```python
from build123d import *

# Parameters (mm, degrees)
SKETCH1_W           = 24.3
SKETCH1_H           = 12.9
BOSS_EXTRUDE1_DEPTH = 51.5
FILLET1_R           = 5
SHELL1_START        = 1.4
SHELL1_DEPTH        = 48.7
SKETCH2_W           = 18.539285396
SKETCH2_H           = 48.7
CUT_EXTRUDE1_DEPTH  = 5
SKETCH3_W           = 24.3
SKETCH3_H           = 4.6
SKETCH3_H_2         = 16.8
CUT_EXTRUDE2_DEPTH  = 5


# Read off the part's stored shape, not the designer's step: Shell1
with BuildPart() as part:
    # Sketch1 → Boss-Extrude1 (new body)
    with BuildSketch(Plane.XY):
        Rectangle(SKETCH1_W, SKETCH1_H)
    extrude(amount=BOSS_EXTRUDE1_DEPTH)

    # Fillet1
    fillet1_edges = [part.edges().sort_by_distance(p)[0] for p in [
        (-12.15, 6.45, 25.75),
        (12.15, 6.45, 25.75),
    ]]
    fillet(fillet1_edges, radius=FILLET1_R)

    # Shell1 outline → Shell1 (cut)
    with BuildSketch(Plane.XY.offset(SHELL1_START)):
        with BuildLine():
            Line((7.15, 5.05), (7.15, 6.45))
            Line((7.15, 6.45), (-7.15, 6.45))
            Line((-7.15, 6.45), (-7.15, 5.05))
            ThreePointArc((-7.15, 5.05), (-9.695584412, 3.995584412), (-10.75, 1.45))
            Line((-10.75, 1.45), (-10.75, -5.05))
            Line((-10.75, -5.05), (10.75, -5.05))
            Line((10.75, -5.05), (10.75, 1.45))
            ThreePointArc((10.75, 1.45), (9.695584412, 3.995584412), (7.15, 5.05))
        make_face()
    extrude(amount=SHELL1_DEPTH, mode=Mode.SUBTRACT)

    # Sketch2 → Cut-Extrude1 (cut)
    with BuildSketch(Plane(origin=(0, 6.45, 0), x_dir=(1, 0, 0), z_dir=(0, 1, 0))):
        with Locations((0, -25.75)):
            Rectangle(SKETCH2_W, SKETCH2_H)
    extrude(amount=-CUT_EXTRUDE1_DEPTH, mode=Mode.SUBTRACT)

    # Sketch3 → Cut-Extrude2 (cut)
    with BuildSketch(Plane(origin=(0, 6.45, 0), x_dir=(1, 0, 0), z_dir=(0, 1, 0))):
        with Locations((0, -3.7)):
            Rectangle(SKETCH3_W, SKETCH3_H)
        with Locations((0, -47.8)):
            Rectangle(SKETCH3_W, SKETCH3_H)
        with Locations((0, -25.75)):
            Rectangle(SKETCH3_W, SKETCH3_H_2)
    extrude(amount=-CUT_EXTRUDE2_DEPTH, mode=Mode.SUBTRACT)


solid = part.part
```
Here's how the part is built. I have some questions about the finished solid (model axes, mm). A direction names the side the tool comes from. Coordinates: 2 decimals unless noted, no trailing zeros. Order: outer loops, then holes, each group sorted by start corner. A loop starts at its lowest first (then second) coordinate and runs counter-clockwise, first axis right, second up.
Item 1: If we section it at B-B, the plane z = 19: List the corners of the cut face in (x, y) for me, then the cut area to 3 significant figures.
Response values:
outline: (-12.15, -6.45) - (12.15, -6.45) - (12.15, 1.45) - (10.75, 1.45) - (10.75, -5.05) - (-10.75, -5.05) - (-10.75, 1.45) - (-12.15, 1.45) - close
area: 52.2 mm2
Item 2: If we section it at A-A, the plane y = -1: List the corners of the cut face in (x, z) for me, then the cut area to 3 significant figures.
Response values:
outline: (-12.15, 0) - (12.15, 0) - (12.15, 51.5) - (-12.15, 51.5) - close; hole (-10.75, 1.4) - (10.75, 1.4) - (10.75, 50.1) - (-10.75, 50.1) - close
area: 204 mm2
Item 3: If we section it at D-D, the plane x = 3.5: List the corners of the cut face in (y, z) for me, then the cut area to 3 significant figures.
Response values:
outline: (-6.45, 0) - (6.45, 0) - (6.45, 1.4) - (-5.05, 1.4) - (-5.05, 50.1) - (6.45, 50.1) - (6.45, 51.5) - (-6.45, 51.5) - close
area: 104 mm2
Item 4: Which directions (+Z, -Z, +X, -X, +Y, -Y) give clear straight access to the entire face, cutting with the end or side of a thin tool? Please do faces 5 (the face through (9.27, 5, 40)), 6 (the face through (11.39, 4.1, 11.75)), 7 (the face through (10.75, -2, 25)), 8 (the face through (11, 4, 6)).
Response values:
face 5: +Y
face 6: +Z, -Z, +X, +Y
face 7: none
face 8: +X, -X, +Y
Item 5: I'm going to push flat-ended pins straight in: pin 1 Ø1 at (x, z) = (-9, 37.5) entering from +Y; pin 2 Ø5 at (y, z) = (4.5, 26) entering from +X; pin 3 Ø1.5 at (x, z) = (11.5, 3.5) entering from +Y; pin 4 Ø10 at (x, z) = (-4.5, 23) entering from +Y. Where does each tip first touch, or does it pass through?
Response values:
pin 1: stops at y = 5.98
pin 2: passes through
pin 3: stops at y = 1.45
pin 4: stops at y = -5.05
Item 6: I need wall thicknesses on probe 1 along Z at (x, y) = (10.5, 3.75); probe 2 along Z at (x, y) = (-9.25, -3.75); probe 3 along X at (y, z) = (-1, 40). Which ranges of each line are inside material? Lowest first, please.
Response values:
probe 1: z = 0 to 1.4, 6 to 17.35, 34.15 to 45.5, 50.1 to 51.5
probe 2: z = 0 to 1.4, 50.1 to 51.5
probe 3: x = -12.15 to -10.75, 10.75 to 12.15
Item 7: If we section it at C-C, the plane y = 3.5: List the corners of the cut face in (x, z) for me, then the cut area to 3 significant figures.
Response values:
outline: (-11.71, 0) - (11.71, 0) - (11.71, 1.4) - (-11.71, 1.4) - close; (-11.71, 6) - (-10.11, 6) - (-10.11, 17.35) - (-11.71, 17.35) - close; (-11.71, 34.15) - (-10.11, 34.15) - (-10.11, 45.5) - (-11.71, 45.5) - close; (-11.71, 50.1) - (11.71, 50.1) - (11.71, 51.5) - (-11.71, 51.5) - close; (10.11, 6) - (11.71, 6) - (11.71, 17.35) - (10.11, 17.35) - close; (10.11, 34.15) - (11.71, 34.15) - (11.71, 45.5) - (10.11, 45.5) - close
area: 138 mm2
Item 8: Thinking about a two-plate mould opening in X: for faces 1 (the face through (0, 1, 1.4)), 2 (the face through (11.39, 4.1, 39.9)), 3 (the face through (-10.72, 4.95, 0.71)), 4 (the face through (-11, 1.45, 48)), which applies, pulls with the +X half, pulls with the -X half, needs draft (parallel to the pull), parting line crosses it, or undercut?
Response values:
face 1: undercut
face 2: pulls with the +X half
face 3: pulls with the -X half
face 4: needs draft
